Verification items for the finished model (mm, model axes). A direction names the side the tool comes from. Give positions to 0.01 mm unless a question says otherwise; leave off trailing zeros. Loops run counter-clockwise (first coordinate to the right, second up) from the corner with the lowest first, then second, coordinate; pieces in that order, holes last. Notation, with made-up numbers: M -16,6.25 L 10,6.25 A14 ccw 10,16.25 Z; hole C 42,53.25 d4. An arc over 180 degrees is marked long. Use a Markdown table: item, result.
from build123d import *

# Parameters (mm, degrees)
F1_DEPTH = 76.2
F2_R     = 27.058381
F3_DEPTH = 27.432
F4_R     = 19.641698
F5_DEPTH = 197.104


with BuildPart() as f1:
    # F0 (on Front) → F1 (new body)
    with BuildSketch(Plane.XZ):
        Polygon((57.671439, 38.690969), (-60.007501, 38.690969), (-60.007501, -43.07108), (57.671439, -43.07108), (57.671439, 35.186879), align=None)
    extrude(amount=-F1_DEPTH)

    # F2 (on Front) → F3 (join)
    with BuildSketch(Plane.XZ):
        Circle(F2_R)
    extrude(amount=F3_DEPTH)

    # F4 (on face) → F5 (cut)
    with BuildSketch(Plane.XZ.offset(27.432)):
        Circle(F4_R)
    extrude(amount=-F5_DEPTH, mode=Mode.SUBTRACT)


solid = f1.part
(1) Material ranges on line 1 (Z direction, x = 0, y = 48); line 2 (X direction, y = 23.5, z = -13); line 3 (Y direction, x = 25, z = 15), recorded low to high.
Results below:
| item | result |
|---|---|
| line 1 | -43.07 to -19.64, 19.64 to 38.69 |
| line 2 | -60.01 to -14.72, 14.72 to 57.67 |
| line 3 | 0 to 76.2 |
(2) Cross-section at C-C on y = 39.5. Record the cut outline in (x, z), then the cut area to 3 significant figures.
Results below:
| item | result |
|---|---|
| outline | M -60.01,-43.07 L 57.67,-43.07 L 57.67,38.69 L -60.01,38.69 Z; hole C 0,0 d39.28 |
| area | 8,410 mm^2 |
(3) Cross-section at A-A on x = 0. Record the cut outline in (y, z), then the cut area to 3 significant figures.
Results below:
| item | result |
|---|---|
| outline | M -27.43,-27.06 L 0,-27.06 L 0,-43.07 L 76.2,-43.07 L 76.2,-19.64 L -27.43,-19.64 Z; M -27.43,19.64 L 76.2,19.64 L 76.2,38.69 L 0,38.69 L 0,27.06 L -27.43,27.06 Z |
| area | 3,640 mm^2 |
(4) Gauge pin test, flat ends, axial feed: P1, Ø1, axis at y = -5.5, z = -23.5, coming from the -X side; P2, Ø3, axis at x = 6.5, y = -16.5, coming from the -Z side; P3, Ø23.5, axis at x = 0, z = 0, coming from the -Y side; P4, Ø5, axis at x = 41, z = 9.5, coming from the -Y side. Record the tip position at first contact, or that the pin passes through.
Results below:
| item | result |
|---|---|
| P1 | x = -14.25 |
| P2 | z = -26.59 |
| P3 | through |
| P4 | y = 0 |
(5) Cross-section at D-D on z = -22.5. Record the cut outline in (x, y).
Results below:
| item | result |
|---|---|
| outline | M -60.01,0 L -15.03,0 L -15.03,-27.43 L 15.03,-27.43 L 15.03,0 L 57.67,0 L 57.67,76.2 L -60.01,76.2 Z |
(6) Draft check along X on faces 1 (the flat face through (-60.008, 38, -2)), 2 (the cylindrical face through (-19.623, 23.659, 0.864)), 3 (the flat face through (-2, 76.2, -20)), 4 (the cylindrical face through (24.995, -13.524, -10.364)). Enter one of: +X half, -X half, draft (parallel to the pull), parting line (faces both ways), or undercut.
Results below:
| item | result |
|---|---|
| face 1 | -X half |
| face 2 | undercut |
| face 3 | draft |
| face 4 | parting line |
(7) Set-up check for faces 5 (the flat face through (14, -27.432, 14)), 6 (the flat face through (-28, 0, -2)): record each of +Z, -Z, +X, -X, +Y, -Y from which the full face is reachable in a straight line by a thin tool's end or side.
Results below:
| item | result |
|---|---|
| face 5 | +Z, -Z, +X, -X, -Y |
| face 6 | -Y |
(8) Cross-section at B-B on z = 0. Record the cut outline in (x, y), then the cut area to 3 significant figures.
Results below:
| item | result |
|---|---|
| outline | M -60.01,0 L -27.06,0 L -27.06,-27.43 L -19.64,-27.43 L -19.64,76.2 L -60.01,76.2 Z; M 19.64,-27.43 L 27.06,-27.43 L 27.06,0 L 57.67,0 L 57.67,76.2 L 19.64,76.2 Z |
| area | 6,380 mm^2 |
